Autodesk Inventor part; units mm, degrees
ref_plane "YZ Plane" through (0, 0, 0) normal (1, 0, 0) x (0, 1, 0)
ref_plane "XZ Plane" through (0, 0, 0) normal (0, 1, 0) x (-1, 0, 0)
ref_plane "XY Plane" through (0, 0, 0) normal (0, 0, 1) x (1, 0, 0)
sketch "Sketch1" plane through (0, 0, 0) normal (0, 1, 0) x (-1, 0, 0)
  arc A0 (13.4296, 151.8071) -> (151.8071, 13.4296) centre (0, 0) ccw
  line L0 (13.4296, 151.8071) -> (151.8071, 13.4296)
  dimension "d0" = 304.8
sketch "Sketch2" plane through (0, 0, 0) normal (0, 1, 0) x (-1, 0, 0)
  line L0 (-4.2626, 135.0266) -> (-129.9862, 9.3031)
  line L1 (-129.9862, 9.3031) -> (13.6979, -134.381)
  line L2 (13.6979, -134.381) -> (139.4215, -8.6575)
  line L3 (139.4215, -8.6575) -> (-4.2626, 135.0266)
  line L4 (-4.2626, 135.0266) -> (-76.1046, 63.1846)
  line L5 (-76.1046, 63.1846) -> (-4.2626, -8.6575)
  line L6 (-4.2626, -8.6575) -> (67.5795, 63.1846)
  line L7 (67.5795, 63.1846) -> (-4.2626, 135.0266)
  line L8 (-129.9862, 9.3031) -> (-76.1046, 63.1846)
  line L9 (-76.1046, 63.1846) -> (-4.2626, -8.6575)
  line L10 (-4.2626, -8.6575) -> (-58.1441, -62.539)
  line L11 (-58.1441, -62.539) -> (-129.9862, 9.3031)
  line L12 (-4.2626, 130.5365) -> (-71.6145, 63.1846)
  line L13 (-71.6145, 63.1846) -> (-4.2626, -4.1673)
  line L14 (-4.2626, -4.1673) -> (63.0893, 63.1846)
  line L15 (63.0893, 63.1846) -> (-4.2626, 130.5365)
  line L16 (-125.496, 9.3031) -> (-76.1046, 58.6945)
  line L17 (-76.1046, 58.6945) -> (-8.7527, -8.6575)
  line L18 (-8.7527, -8.6575) -> (-58.1441, -58.0489)
  line L19 (-58.1441, -58.0489) -> (-125.496, 9.3031)
  line L20 (67.5795, 58.6945) -> (-53.654, -62.539)
  line L21 (-53.654, -62.539) -> (13.6979, -129.8909)
  line L22 (13.6979, -129.8909) -> (134.9314, -8.6575)
  line L23 (134.9314, -8.6575) -> (67.5795, 58.6945)
  point P0 (0, 0)
  point P1 (4.7177, 0.3228)
  dimension "d42" = 203.2
  dimension "d43" = 177.8
  dimension "d44" = 3.175
  dimension "d45" = 6.35
  dimension "d46" = 95.25
  dimension "d47" = 171.45
  dimension "d48" = 95.25
  dimension "d49" = 69.85
  dimension "d50" = 95.25
extrude "Extrusion1" add sketch "Sketch1" against normal blind 12.7
extrude "Extrusion2" add sketch "Sketch2" along normal blind 127
sketch "Sketch3" plane through (-13.6979, 0, -134.381) normal (0.7071068, 0, -0.7071068) x (-0.7071068, 0, -0.7071068)
  line L0 (-29.972, 4.7625) -> (-71.628, 4.7625)
  line L1 (-74.803, 7.9375) -> (-74.803, 49.5935)
  line L2 (-71.628, 52.7685) -> (-29.972, 52.7685)
  line L3 (-26.797, 49.5935) -> (-26.797, 7.9375)
  line L4 (-257.1076, 0) -> (47.6924, 0)
  line L5 (0, 0) -> (0, 127)
  arc A0 (-26.797, 49.5935) -> (-29.972, 52.7685) centre (-29.972, 49.5935) ccw
  arc A1 (-29.972, 4.7625) -> (-26.797, 7.9375) centre (-29.972, 7.9375) ccw
  arc A2 (-74.803, 7.9375) -> (-71.628, 4.7625) centre (-71.628, 7.9375) ccw
  arc A3 (-71.628, 52.7685) -> (-74.803, 49.5935) centre (-71.628, 49.5935) ccw
  point P0 (-104.7076, 0)
  point P1 (-74.803, 52.7685)
  point P2 (-74.803, 4.7625)
  point P3 (-26.797, 52.7685)
  point P4 (-6.8599, 0)
  point P5 (-202.5554, 0)
  dimension "d25" = 4.7625
  dimension "d26" = 48.006
  dimension "d27" = 26.797
  dimension "d28" = 48.006
  dimension "d29" = 3.175
sketch "Sketch4" plane through (4.2626, 0, 135.0266) normal (-0.7071068, 0, 0.7071068) x (0.7071068, 0, 0.7071068)
  line L0 (-98.425, 52.7812) -> (-50.419, 52.7812)
  line L1 (-50.419, 52.7812) -> (-50.419, 4.7752)
  line L2 (-50.419, 4.7752) -> (-98.425, 4.7752)
  line L3 (-98.425, 4.7752) -> (-98.425, 52.7812)
  line L4 (-0.6446, 0) -> (-196.3401, 0)
  line L5 (0, 0) -> (0, 127)
  point P0 (-98.4924, 0)
  dimension "d30" = 48.006
  dimension "d31" = 48.006
  dimension "d32" = 4.7752
  dimension "d33" = 50.419
extrude "Extrusion3" cut sketch "Sketch4" against normal up to next
extrude "Extrusion4" cut sketch "Sketch3" against normal up to next
sketch "Sketch5" plane through (0, 127, 0) normal (0, 1, 0) x (1, 0, 0)
  line L0 (-139.4215, 8.6575) -> (-13.6979, 134.381)
  line L1 (4.2626, -135.0266) -> (-139.4215, 8.6575)
  line L2 (-139.4215, 8.6575) -> (-13.6979, 134.381)
  line L3 (-13.6979, 134.381) -> (129.9862, -9.3031)
  line L4 (-13.6979, 134.381) -> (129.9862, -9.3031)
  line L5 (129.9862, -9.3031) -> (4.2626, -135.0266)
  point P0 (0, 0)
extrude "Extrusion5" cut sketch "Sketch5" against normal blind 3.175
sketch "Sketch6" plane through (0, 123.825, 0) normal (0, 1, 0) x (1, 0, 0)
  line L0 (4.2626, -135.0266) -> (-139.4215, 8.6575)
  line L1 (4.2626, -135.0266) -> (-139.4215, 8.6575)
  line L2 (-139.4215, 8.6575) -> (-13.6979, 134.381)
  line L3 (-13.6979, 134.381) -> (129.9862, -9.3031)
  line L4 (-13.6979, 134.381) -> (129.9862, -9.3031)
  line L5 (129.9862, -9.3031) -> (4.2626, -135.0266)
  line L6 (4.2626, -130.5365) -> (71.6145, -63.1846)
  point P0 (0, 0)
extrude "Extrusion6" add sketch "Sketch6" along normal blind 3.175
sketch "Sketch7" plane through (0, 127, 0) normal (0, 1, 0) x (1, 0, 0)
  point P0 (0, 0)
properties part number "Hermes plate" material "Aluminum 6061"
Design review of the part built by this model. Coordinates are the model's own, in mm. A direction names the side the tool comes from. Round coordinates to 2 decimals unless told otherwise and drop trailing zeros. Write each loop counter-clockwise with the first axis right and the second up, starting at its lowest first coordinate (ties: lowest second). Pieces come first, ordered by that corner, then holes.
Item 1: Wall thickness on L1, parallel to Y at x = 57, z = 21 (3 decimals); L2, parallel to Z at x = -19.5, y = 81 (3 decimals); L3, parallel to Z at x = 9, y = 20.5 (3 decimals): over which ranges is each line inside the solid? List them lowest first.
Item 2: Draft analysis for pull direction Z (two halves, no side actions). For faces 5 (the flat face through (57.138, 62.611, -63.545)), 6 (the flat face through (-7.811, 61.046, -1.074)), 7 (the flat face through (38.41, 61.05, 29.98)), 8 (the flat face through (-7, 127, -2)), state which applies: released by +Z, released by -Z, zero draft, split by the parting line, or undercut.
Item 3: Consider section C-C on z = 0. Give the boundary of the cut face in (x, y) (3 decimals), and give its area (3 significant figures).
Item 4: For faces 1 (the flat face through (101.1, 61, 33.7)), 2 (the flat face through (68.004, 62.611, 71.285)), 3 (the flat face through (-66.574, 62.611, 64.19)), 4 (the flat face through (70, 0, -66)), list the 3-axis set-ups (+Z, -Z, +X, -X, +Y, -Y) from which the entire face can be reached by the end or side of a thin tool; tool diameter is ignored.
Item 5: Consider section B-B on z = -92. Give the boundary of the cut face in (x, y) (1 decimal).
Item 6: For pin 1 Ø3 at (y, z) = (48, 36) entering from +X; pin 2 Ø1.5 at (y, z) = (85.5, -70) entering from +X; pin 3 Ø8 at (x, y) = (-101, 47) entering from +Z; pin 4 Ø11 at (x, z) = (-53, 78.5) entering from +Y, all flat-tipped, find the tip position at first contact; note any pin that passes through.
Item 7: Consider section D-D on z = 46. Give the boundary of the cut face in (x, y) (3 decimals).
Item 8: Consider section A-A on x = 18.5. Give the boundary of the cut face in (y, z) (1 decimal).
Check values:
1. L1: y = -12.7 to 0, 123.825 to 127
1. L2: z = -128.579 to -124.089, 10.615 to 19.595, 106.774 to 111.264
1. L3: z = -17.885 to -8.905, -8.41 to 0.57, 125.799 to 130.289
2. face 5: released by -Z
2. face 6: undercut
2. face 7: undercut
2. face 8: zero draft
3. outline: (-152.4, -12.7) - (152.4, -12.7) - (152.4, 0) - (120.683, 0) - (120.683, 127) - (-130.764, 127) - (-130.764, 0) - (-152.4, 0) - close; hole (-126.274, 0) - (-8.885, 0) - (-8.885, 123.825) - (-126.274, 123.825) - close; hole (0.095, 0) - (8.43, 0) - (8.43, 123.825) - (0.095, 123.825) - close; hole (17.41, 0) - (116.193, 0) - (116.193, 123.825) - (17.41, 123.825) - close
3. area: 8,010 mm2
4. face 1: none
4. face 2: +Z, +X, +Y
4. face 3: +Z, -X, +Y
4. face 4: +Y
5. outline: (-121.5, -12.7) - (121.5, -12.7) - (121.5, 0) - (28.7, 0) - (28.7, 4.8) - (24.2, 4.8) - (24.2, 0) - (-51.6, 0) - (-51.6, 123.8) - (24.2, 123.8) - (24.2, 52.8) - (28.7, 52.8) - (28.7, 127) - (-56.1, 127) - (-56.1, 0) - (-121.5, 0) - close
6. pin 1: stops at x = 104.79
6. pin 2: stops at x = 51.43
6. pin 3: stops at z = 33.76
6. pin 4: stops at y = 127
7. outline: (-119.237, -12.7) - (145.292, -12.7) - (145.292, 0) - (93.289, 0) - (93.289, 127) - (-84.764, 127) - (-84.764, 0) - (-119.237, 0) - close; hole (-80.274, 0) - (-54.885, 0) - (-54.885, 123.825) - (-80.274, 123.825) - close; hole (-45.905, 0) - (54.43, 0) - (54.43, 123.825) - (-45.905, 123.825) - close; hole (63.41, 0) - (88.799, 0) - (88.799, 123.825) - (63.41, 123.825) - close
8. outline: (-12.7, -151.3) - (0, -151.3) - (0, -102.2) - (4.8, -102.2) - (4.8, -97.7) - (0, -97.7) - (0, -27.4) - (123.8, -27.4) - (123.8, -97.7) - (52.8, -97.7) - (52.8, -102.2) - (127, -102.2) - (127, 120.8) - (0, 120.8) - (0, 151.3) - (-12.7, 151.3) - close; hole (0, -18.4) - (123.8, -18.4) - (123.8, 1.1) - (0, 1.1) - close; hole (0, 10.1) - (123.8, 10.1) - (123.8, 116.3) - (0, 116.3) - close
